Design review of the part built by this model. Coordinates are the model's own, in mm. A direction names the side the tool comes from. Coordinates: 2 decimals unless noted, no trailing zeros. Order: outer loops, then holes, each group sorted by start corner. A loop starts at its lowest first (then second) coordinate and runs counter-clockwise, first axis right, second up. Notation, with made-up numbers: (10, -23) -> (59, -23) arc R37 ccw to (59, 14) -> close; hole circle Ø4 at (-18.75, -22). An arc over 180 degrees is marked (long way). Write item = value, one per line.
```python
from build123d import *

# Parameters (mm, degrees)
SKETCH_1_W           = 54.61
SKETCH_1_H           = 29.97
EXTRUDE_1_DEPTH      = 2.5
EXTRUDE_2_DEPTH      = 17
CUT_EXTRUDE_1_DEPTH  = 30.97
EXTRUDE_4_DEPTH      = 9.5
EXTRUDE_4_DEPTH_BACK = 9.5
SKETCH_10_R          = 3.75
EXTRUDE_6_DEPTH      = 1
SKETCH_11_R          = 3
SKETCH_11_R_2        = 2
EXTRUDE_7_DEPTH      = 4
SKETCH_12_R          = 4.25
SKETCH_12_R_2        = 3.25
EXTRUDE_8_DEPTH      = 4


with BuildPart() as part:
    # Эскиз1 → Бобышка-Вытянуть1 (new body)
    with BuildSketch(Plane(origin=(0, 0, 0), x_dir=(1, 0, 0), z_dir=(0, 1, 0))):
        Rectangle(SKETCH_1_W, SKETCH_1_H)
    extrude(amount=EXTRUDE_1_DEPTH)

    # Эскиз2 → Бобышка-Вытянуть2 (add)
    with BuildSketch(Plane(origin=(0, 2.5, 0), x_dir=(1, 0, 0), z_dir=(0, 1, 0))):
        with BuildLine():
            Line((27.305, -14.985), (-0.695, -14.985))
            Line((-0.695, -14.985), (-0.695, -13.485))
            Line((-0.695, -13.485), (23.305, -13.485))
            ThreePointArc((23.305, -13.485), (24.719213562, -12.899213562), (25.305, -11.485))
            Line((25.305, -11.485), (25.305, 11.485))
            ThreePointArc((25.305, 11.485), (24.719213562, 12.899213562), (23.305, 13.485))
            Line((23.305, 13.485), (-0.695, 13.485))
            Line((-0.695, 13.485), (-0.695, 14.985))
            Line((-0.695, 14.985), (27.305, 14.985))
            Line((27.305, 14.985), (27.305, -14.985))
        make_face()
    extrude(amount=EXTRUDE_2_DEPTH)

    # Эскиз3 → Вырез-Вытянуть1 (cut, through all)
    with BuildSketch(Plane.XY.offset(14.985)):
        Polygon((-0.695, 2.5), (25.305, 19.5), (-0.695, 19.5), align=None)
    extrude(amount=-CUT_EXTRUDE_1_DEPTH, mode=Mode.SUBTRACT)

    # Эскиз8 → Бобышка-Вытянуть4 (add, two sides)
    with BuildSketch(Plane.XY) as extrude_4_sk:
        Polygon((-27.305, 2.5), (-24.695, 13.85), (-23.695, 11.232050808), (-24.695, 9.5), (-24.695, 2.5), align=None)
    extrude(amount=EXTRUDE_4_DEPTH)
    extrude(extrude_4_sk.sketch, amount=-EXTRUDE_4_DEPTH_BACK)

    # Эскиз10 → Бобышка-Вытянуть6 (add)
    with BuildSketch(Plane.ZY.offset(-25.305)):
        with Locations((-6.35, 11.48)):
            Circle(SKETCH_10_R)
        with Locations((6.35, 11.48)):
            Circle(SKETCH_10_R)
    extrude(amount=EXTRUDE_6_DEPTH)

    # Эскиз11 → Бобышка-Вытянуть7 (add)
    with BuildSketch(Plane.ZY.offset(-24.305)):
        with Locations((-6.35, 11.48)):
            Circle(SKETCH_11_R)
        with Locations((-6.35, 11.48)):
            Circle(SKETCH_11_R_2, mode=Mode.SUBTRACT)
    extrude(amount=EXTRUDE_7_DEPTH)

    # Эскиз12 → Бобышка-Вытянуть8 (add)
    with BuildSketch(Plane.ZY.offset(-24.305)):
        with Locations((6.35, 11.48)):
            Circle(SKETCH_12_R)
        with Locations((6.35, 11.48)):
            Circle(SKETCH_12_R_2, mode=Mode.SUBTRACT)
    extrude(amount=EXTRUDE_8_DEPTH)


solid = part.part
```
(1) We need section B-B (x = 4). Write out the cut boundary in (y, z) (3 decimals), and give its area (3 significant figures).
Report:
outline = (0, -14.985) -> (5.57, -14.985) -> (5.57, -13.485) -> (2.5, -13.485) -> (2.5, 13.485) -> (5.57, 13.485) -> (5.57, 14.985) -> (0, 14.985) -> close
area = 84.1 mm²
(2) We need section D-D (z = -5.75). Write out the cut boundary in (x, y) (3 decimals), and give its area (3 significant figures).
Report:
outline = (-27.305, 0) -> (27.305, 0) -> (27.305, 19.5) -> (25.305, 19.5) -> (25.305, 15.182) -> (24.305, 15.182) -> (24.305, 14.419) -> (20.305, 14.419) -> (20.305, 13.388) -> (24.305, 13.388) -> (24.305, 9.572) -> (20.305, 9.572) -> (20.305, 8.541) -> (24.305, 8.541) -> (24.305, 7.778) -> (25.305, 7.778) -> (25.305, 2.5) -> (-24.695, 2.5) -> (-24.695, 9.5) -> (-23.695, 11.232) -> (-24.695, 13.85) -> (-27.305, 2.5) -> close
area = 203 mm²
(3) We need section A-A (z = 6.35). Write out the cut boundary in (x, y) (3 decimals).
Report:
outline = (-27.305, 0) -> (27.305, 0) -> (27.305, 19.5) -> (25.305, 19.5) -> (25.305, 15.23) -> (24.305, 15.23) -> (24.305, 15.73) -> (20.305, 15.73) -> (20.305, 14.73) -> (24.305, 14.73) -> (24.305, 8.23) -> (20.305, 8.23) -> (20.305, 7.23) -> (24.305, 7.23) -> (24.305, 7.73) -> (25.305, 7.73) -> (25.305, 2.5) -> (-24.695, 2.5) -> (-24.695, 9.5) -> (-23.695, 11.232) -> (-24.695, 13.85) -> (-27.305, 2.5) -> close
(4) The part is to be moulded in two halves that separate along X. For faces 1 (the flat face through (10, 6, -14.985)), 2 (the flat face through (27.305, 10, 0)), 3 (the flat face through (20.305, 11, -4)), 4 (the flat face through (-24.188, 10.378, 0.133)), say which applies: released by +X, released by -X, zero draft, split by the parting line, or undercut.
Report:
face_1 = zero draft
face_2 = released by +X
face_3 = undercut
face_4 = undercut
(5) For faces 5 (the flat face through (-25, 7, 9.5)), 6 (the flat face through (16, 7, 13.485)), 7 (the flat face through (-25, 7, -9.5)), 8 (the flat face through (-24.695, 6, 0)), 9 (the flat face through (25.305, 11, 0)), list the 3-axis set-ups (+Z, -Z, +X, -X, +Y, -Y) from which the entire face can be reached by the end or side of a thin tool; tool diameter is ignored.
Report:
face_5 = +Z, -X, +Y
face_6 = -X, +Y
face_7 = -Z, -X, +Y
face_8 = +Z, -Z
face_9 = none
(6) We need section C-C (z = 0). Write out the cut boundary in (x, y) (3 decimals).
Report:
outline = (-27.305, 0) -> (27.305, 0) -> (27.305, 19.5) -> (25.305, 19.5) -> (25.305, 2.5) -> (-24.695, 2.5) -> (-24.695, 9.5) -> (-23.695, 11.232) -> (-24.695, 13.85) -> (-27.305, 2.5) -> close
(7) Insertion check: pin 1 (8.5 mm diameter, centred on y = 7.5, z = -4, fed in from -X); pin 2 (2 mm diameter, centred on y = 12, z = -6.5, fed in from -X); pin 3 (1.5 mm diameter, centred on y = 16.5, z = 2.5, fed in from -X) (3 decimals). Each pin has a flat end and moves straight along its axis. Give the tip position at first contact, or say it passes through.
Report:
pin_1 = -27.13
pin_2 = -25.35
pin_3 = 25.305
(8) For L1, parallel to Y at x = 22.95, z = -6.35; L2, parallel to Y at x = 23.15, z = 6.35; L3, parallel to Y at x = -15.5, z = 3.75, list the stretches that pass through material, from the lowest coordinate up.
Report:
L1 = 0 to 2.5, 8.48 to 9.48, 13.48 to 14.48
L2 = 0 to 2.5, 7.23 to 8.23, 14.73 to 15.73
L3 = 0 to 2.5
